For this review, take the finished solid that the model builds, in its own axes (mm). Face numbers are marked on the shaded views. A direction names the side the tool comes from. Coordinates: 2 decimals unless noted, no trailing zeros. Write each loop counter-clockwise with the first axis right and the second up, starting at its lowest first coordinate (ties: lowest second). Pieces come first, ordered by that corner, then holes. Notation, with made-up numbers: (-30, 39.5) -> (-10, 39.5) arc R22 cw to (-10, 58.5) -> close; hole circle Ø5 at (23, -40). An arc over 180 degrees is marked (long way). One line per item, written item: value. Start each with the question number.
1) Add section C-C (y = -10.75). State the section outline as (x, z) points.
2) Add section B-B (x = 31). State the section outline as (y, z) points.
3) Mouldability with a two-part tool opening along X and no side actions: class the marked faces 1, 2 and 3 as released by +X, released by -X, zero draft, split by the parting line, or undercut.
4) Machinability: for the marked faces 4 and 5, which of the approach directions +Z, -Z, +X, -X, +Y, -Y give a long, thin tool a straight path to every point of the face, cutting with its end or side? Answer none if there is none.
5) Add section A-A (x = 2). State the section outline as (y, z) points, and give its area (3 significant figures).
6) For pin 1 Ø2 at (x, y) = (32, -6.5) entering from -Z; pin 2 Ø10 at (y, z) = (-16.5, 21.5) entering from -X; pin 3 Ø2 at (x, y) = (-10, -21) entering from -Z, all flat-tipped, find the tip position at first contact; note any pin that passes through.
7) Add section D-D (z = 27.5). State the section outline as (x, y) points, and give its area (3 significant figures).
8) For probe 1 along Z at (x, y) = (39, -4.5); probe 2 along Z at (x, y) = (35, -12.75); probe 3 along X at (y, z) = (-13.5, 60), list the stretches that pass through material, from the lowest coordinate up. Write a range as from..to.
from build123d import *

# Parameters (mm, degrees)
F0_R     = 5.227515474
F1_DEPTH = 25.4
F2_DEPTH = 25.4


# Not quite as in the source:
# - a feature names something its author has since deleted; it is built from what else it names


with BuildPart() as f1:
    # F0 (on Front) → F1 (new body)
    with BuildSketch(Plane.XZ):
        with BuildLine():
            Line((0, 0), (48.4997071326, 16.699001193))
            ThreePointArc((48.4997071326, 16.699001193), (33.4463476719, 38.6685413288), (9.4887581342, 50.3003179933))
            ThreePointArc((9.4887581342, 50.3003179933), (0.0976286062, 69.1824149389), (-9.603985867, 50.457950314))
            ThreePointArc((-9.603985867, 50.457950314), (-39.5504687593, -35.0093012615), (49.08054322, -16.408585012))
            Line((49.08054322, -16.408585012), (0, 0))
        make_face()
        with Locations((0, 60.5520345271)):
            Circle(F0_R, mode=Mode.SUBTRACT)
    extrude(amount=F1_DEPTH)

    # F0 (on Front) → F2 (join)
    with BuildSketch(Plane.XZ):
        with BuildLine():
            Line((0, 0), (48.4997071326, 16.699001193))
            ThreePointArc((48.4997071326, 16.699001193), (33.4463476719, 38.6685413288), (9.4887581342, 50.3003179933))
            ThreePointArc((9.4887581342, 50.3003179933), (0.0976286062, 69.1824149389), (-9.603985867, 50.457950314))
            ThreePointArc((-9.603985867, 50.457950314), (-39.5504687593, -35.0093012615), (49.08054322, -16.408585012))
            Line((49.08054322, -16.408585012), (0, 0))
        make_face()
        with Locations((0, 60.5520345271)):
            Circle(F0_R, mode=Mode.SUBTRACT)
    extrude(amount=F2_DEPTH)


solid = f1.part
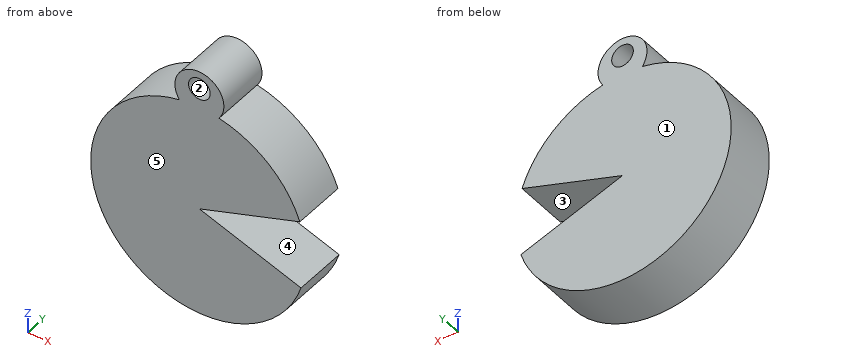
Numbers:
1. outline: (-9.6, 50.46) arc R51.98 ccw (long way) to (49.08, -16.41) -> (0, 0) -> (48.5, 16.7) arc R51.98 ccw to (9.49, 50.3) arc R11.83 ccw (long way) to start; hole circle Ø10.46 at (0, 60.55)
2. outline: (-25.4, -42.09) -> (0, -42.09) -> (0, -10.36) -> (-25.4, -10.36) -> close; (-25.4, 10.67) -> (0, 10.67) -> (0, 40.65) -> (-25.4, 40.65) -> close
3. face 1: zero draft
3. face 2: undercut
3. face 3: released by +X
4. face 4: +X, +Y, -Y
4. face 5: +Z, -Z, +X, -X, -Y
5. outline: (-25.4, -52.64) -> (0, -52.64) -> (0, -0.67) -> (-25.4, -0.67) -> close; (-25.4, 0.69) -> (0, 0.69) -> (0, 55.72) -> (-25.4, 55.72) -> close; (-25.4, 65.38) -> (0, 65.38) -> (0, 69.01) -> (-25.4, 69.01) -> close
5. area: 2,810 mm²
6. pin 1: z = -42.09
6. pin 2: x = -49.53
6. pin 3: z = -52
7. outline: (-44.14, -25.4) -> (43.18, -25.4) -> (43.18, 0) -> (-44.14, 0) -> close
7. area: 2,220 mm²
8. probe 1: -34.54..-13.04, 13.43..33.1
8. probe 2: -38.71..-11.7, 12.05..37.28
8. probe 3: -11.53..-5.2, 5.2..11.53
